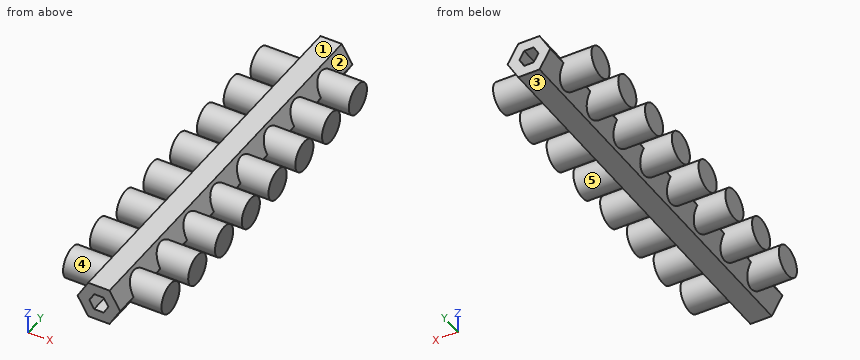
Autodesk Inventor part; units mm, degrees
ref_plane "YZ Plane" through (0, 0, 0) normal (1, 0, 0) x (0, 1, 0)
ref_plane "XZ Plane" through (0, 0, 0) normal (0, 1, 0) x (-1, 0, 0)
ref_plane "XY Plane" through (0, 0, 0) normal (0, 0, 1) x (1, 0, 0)
sketch "Outer Diameter Sketch" plane through (0, 0, 0) normal (0, 1, 0) x (-1, 0, 0)
  line L0 (0, -28.0163) -> (0, 28.3344) construction
  line L1 (17.1062, 0) -> (-23.8822, 0) construction
  line L2 (3.4641, -6) -> (6.9282, 0)
  line L3 (6.9282, 0) -> (3.4641, 6)
  line L4 (3.4641, 6) -> (-3.4641, 6)
  line L5 (-3.4641, 6) -> (-6.9282, 0)
  line L6 (-6.9282, 0) -> (-3.4641, -6)
  line L7 (-3.4641, -6) -> (3.4641, -6)
  line L8 (0, -6) -> (0, 6) construction
  line L9 (-6.9282, 0) -> (6.9282, 0) construction
  point P0 (0, 0)
  dimension "d23" = 120
  dimension "d25" = 120
  dimension "d27" = 120
  dimension "d29" = 120
  dimension "d31" = 120
  dimension "d32" = 12
extrude "Outer Diameter Extrusion" add sketch "Outer Diameter Sketch" along normal mid plane 128
sketch "Sketch2" plane through (0, 0, 0) normal (1, 0, 0) x (0, 1, 0)
  circle A0 centre (-7.375, 0) radius 5
  line L0 (-71.375, 0) -> (-7.375, 0) construction
  line L1 (-7.375, 0) -> (56.625, 0) construction
  circle A1 centre (7.375, 0) radius 5
  circle A2 centre (22.125, 0) radius 5
  circle A3 centre (36.875, 0) radius 5
  circle A4 centre (-22.125, 0) radius 5
  circle A5 centre (-7.375, 0) radius 5
  circle A6 centre (7.375, 0) radius 5
  circle A7 centre (22.125, 0) radius 5
  circle A8 centre (-36.875, 0) radius 5
  circle A9 centre (-22.125, 0) radius 5
  circle A10 centre (-7.375, 0) radius 5
  circle A11 centre (7.375, 0) radius 5
  circle A12 centre (-51.625, 0) radius 5
  circle A13 centre (-36.875, 0) radius 5
  circle A14 centre (-22.125, 0) radius 5
  circle A15 centre (-7.375, 0) radius 5
  line L2 (0, 54.0285) -> (0, -72.3739) construction
  circle A16 centre (51.625, 0) radius 5
  circle A17 centre (36.875, 0) radius 5
  circle A18 centre (22.125, 0) radius 5
  circle A19 centre (7.375, 0) radius 5
  dimension "d3" = 10
  dimension "d5" = 128
  dimension "d8" = 14.75
  dimension "d11" = 14.75
  dimension "d47" = 7.375
  dimension "d48" = 7.375
extrude "Peg Extrusions" add sketch "Sketch2" along normal mid plane 32
sketch "Sketch3" plane through (0, -64, 0) normal (0, -1, 0) x (1, 0, 0)
  line L0 (1.55, -2.6847) -> (-1.55, -2.6847)
  line L1 (-1.55, -2.6847) -> (-3.1, 0)
  line L2 (-3.1, 0) -> (-1.55, 2.6847)
  line L3 (-1.55, 2.6847) -> (1.55, 2.6847)
  line L4 (1.55, 2.6847) -> (3.1, 0)
  line L5 (3.1, 0) -> (1.55, -2.6847)
  line L6 (3.1, 0) -> (-3.1, 0) construction
  line L7 (0, 2.6847) -> (0, -2.6847) construction
  line L8 (10.3659, 0) -> (-11.745, 0) construction
  line L9 (0, -9.4896) -> (0, 9.303) construction
  point P0 (0, 0)
  dimension "d33" = 3.1
  dimension "d34" = 3.1
  dimension "d35" = 120
  dimension "d36" = 3.1
  dimension "d37" = 120
  dimension "d38" = 3.1
  dimension "d39" = 120
  dimension "d40" = 3.1
  dimension "d41" = 120
extrude "Inner Hex Cut" cut sketch "Sketch3" against normal up to surface (128 mm away)
equation "\"d1\" = outL"
equation "\"d3\" = pegD"
equation "\"d5\" = outL"
equation "\"d47\" = 0.5 * d8"
equation "\"d14\" = pegL + 2 * outD"
equation "\"d33\" = inhexSL"
equation "\"d34\" = inhexSL"
equation "\"d36\" = inhexSL"
equation "\"d38\" = inhexSL"
equation "\"d40\" = inhexSL"
equation "\"d42\" = pegL + 2 * outD"
equation "\"outD\" = 12"
equation "\"inhexSL\" = 3.1"
equation "\"outL\" = 128"
equation "\"pegL\" = 8"
equation "\"pegD\" = 10"
equation "\"outhexSL\" = 5"
properties part number "Peg Spinner V4"
Could you check a few things on this model? Use its own coordinates, in mm. Face numbers are marked on the shaded views. A direction names the side the tool comes from. Round coordinates to 2 decimals unless told otherwise and drop trailing zeros. Loops run counter-clockwise (first coordinate to the right, second up) from the corner with the lowest first, then second, coordinate; pieces in that order, holes last. Notation, with made-up numbers: M -15.5,58.25 L -3.5,58.25 A17 cw -3.5,64.25 Z; hole C 36.5,0 d9. An arc over 180 degrees is marked long. Put each result on its own line as item: value.
Q1. I need wall thicknesses on probe 1 along Z at (x, y) = (-1.5, 6); probe 2 along X at (y, z) = (58.5, 1.25); probe 3 along X at (y, z) = (-44, -2.5). Which ranges of each line are inside material? Lowest first, please.
Check result:
probe 1: -6 to -2.68, 2.68 to 6
probe 2: -6.21 to -2.38, 2.38 to 6.21
probe 3: -5.48 to -1.66, 1.66 to 5.48
Q2. Imagine slicing it at A-A (y = 0). Write out the boundary of the cut face in (x, z).
Check result:
outline: M -6.93,0 L -3.46,-6 L 3.46,-6 L 6.93,0 L 3.46,6 L -3.46,6 Z; hole M -3.1,0 L -1.55,-2.68 L 1.55,-2.68 L 3.1,0 L 1.55,2.68 L -1.55,2.68 Z
Q3. For pin 1 (1 mm diameter, centred on x = 4, y = -39.5, fed in from +Z); pin 2 (4 mm diameter, centred on x = 11.5, z = 0.5, fed in from +Y) (3 decimals); pin 3 (3 mm diameter, centred on x = -12, y = 34.5, fed in from +Z), each with a flat end and sliding along its axis, tell me the tip position at first contact or that it passes through.
Check result:
pin 1: z = 5.94
pin 2: y = 56.625
pin 3: z = 4.92
Q4. On a 3-axis mill with a long thin cutter (end or side, diameter ignored), from which of +Z, -Z, +X, -X, +Y, -Y can I reach the whole of each face in a straight line? I mean the marked faces 3, 4 and 5. Say none if no direction works.
Check result:
face 3: -Z, +X, -X, +Y, -Y
face 4: -X
face 5: +X
Q5. Thinking about a two-plate mould opening in Y: for the marked faces 1 and 2, which applies, released by +Y, released by -Y, zero draft, split by the parting line, or undercut?
Check result:
face 1: zero draft
face 2: undercut
Q6. Imagine slicing it at B-B (y = 34). Write out the boundary of the cut face in (x, z).
Check result:
outline: M -16,-4.09 L -4.57,-4.09 L -3.46,-6 L 3.46,-6 L 4.57,-4.09 L 16,-4.09 L 16,4.09 L 4.57,4.09 L 3.46,6 L -3.46,6 L -4.57,4.09 L -16,4.09 Z; hole M -3.1,0 L -1.55,-2.68 L 1.55,-2.68 L 3.1,0 L 1.55,2.68 L -1.55,2.68 Z
